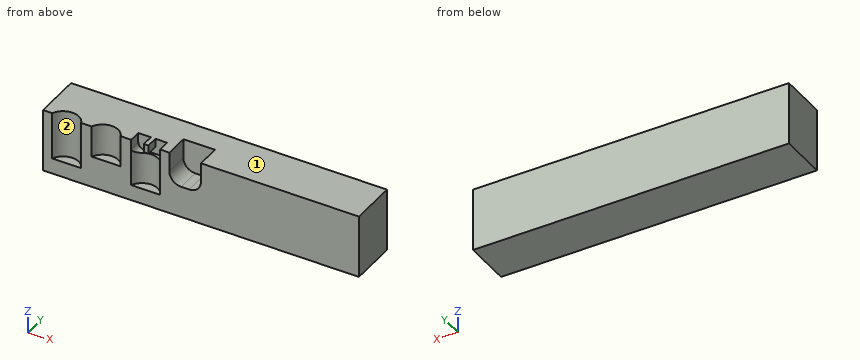
from build123d import *

# Parameters (mm, degrees)
F0_W      = 38.1
F0_H      = 50.8
F1_DEPTH  = 254
F3_DEPTH  = 38.1
F5_DEPTH  = 25.4
F7_DEPTH  = 38.1
F8_W      = 23.2794845304
F8_H      = 9.0677170083
F8_H_2    = 9.5680775121
F9_DEPTH  = 12.7
F10_R     = 5.08
F11_W     = 3.6223009229
F11_H     = 6.850992012
F12_DEPTH = 9.525
F14_DEPTH = 19.05
F15_R     = 9.525


with BuildPart() as f1:
    # F0 (on Right) → F1 (new body)
    with BuildSketch(Plane.YZ):
        with Locations((19.05, 25.4)):
            Rectangle(F0_W, F0_H)
    extrude(amount=F1_DEPTH)

    # F2 (on face) → F3 (cut)
    with BuildSketch(Plane.XY.offset(50.8)):
        with BuildLine():
            ThreePointArc((6.35, -5.08), (19.05, -17.78), (31.75, -5.08))
            ThreePointArc((31.75, -5.08), (19.05, 7.62), (6.35, -5.08))
        make_face()
    extrude(amount=-F3_DEPTH, mode=Mode.SUBTRACT)

    # F4 (on face) → F5 (cut)
    with BuildSketch(Plane.XY.offset(50.8)):
        with BuildLine():
            ThreePointArc((38.1, -5.08), (50.8, -17.78), (63.5, -5.08))
            ThreePointArc((63.5, -5.08), (50.8, 7.62), (38.1, -5.08))
        make_face()
    extrude(amount=-F5_DEPTH, mode=Mode.SUBTRACT)

    # F6 (on face) → F7 (cut)
    with BuildSketch(Plane.XY.offset(50.8)):
        with BuildLine():
            ThreePointArc((69.85, -5.08), (82.55, -17.78), (95.25, -5.08))
            ThreePointArc((95.25, -5.08), (82.55, 7.62), (69.85, -5.08))
        make_face()
    extrude(amount=-F7_DEPTH, mode=Mode.SUBTRACT)

    # F8 (on face) → F9 (cut)
    with BuildSketch(Plane.XY.offset(50.8)):
        with Locations((82.55, -4.5338585041)):
            Rectangle(F8_W, F8_H)
        with Locations((82.55, 4.784038756)):
            Rectangle(F8_W, F8_H_2)
    extrude(amount=-F9_DEPTH, mode=Mode.SUBTRACT)

    # F10
    f10_edges = [f1.edges().sort_by_distance(p)[0] for p in [
        (70.910258, 4.784039, 38.1),
        (94.189742, 4.784039, 38.1),
    ]]
    fillet(f10_edges, radius=F10_R)

    # F11 (on face) → F12 (join)
    with BuildSketch(Plane.XZ.offset(-9.5680775121)):
        with Locations((82.8721560538, 47.374503994)):
            Rectangle(F11_W, F11_H)
    extrude(amount=F12_DEPTH)

    # F13 (on face) → F14 (cut)
    with BuildSketch(Plane.XZ):
        Polygon((101.6, 50.8), (101.6, 38.1), (101.6, 25.4), (127, 25.4), (127, 50.8), align=None)
    extrude(amount=-F14_DEPTH, mode=Mode.SUBTRACT)

    # F15
    f15_edges = [f1.edges().sort_by_distance(p)[0] for p in [
        (101.6, 9.525, 25.4),
        (127, 9.525, 25.4),
    ]]
    fillet(f15_edges, radius=F15_R)


solid = f1.part
Geometry check sheet. Reference: the model listing, model coordinates, mm. Face numbers are marked on the shaded views. A direction names the side the tool comes from. Round coordinates to 2 decimals unless told otherwise and drop trailing zeros. Loops run counter-clockwise (first coordinate to the right, second up) from the corner with the lowest first, then second, coordinate; pieces in that order, holes last. Notation, with made-up numbers: (-11.5, 17) -> (32.5, 17) arc R18 ccw to (32.5, 48) -> close; hole circle Ø7 at (-31.5, 24.25). An arc over 180 degrees is marked (long way). Answer as a JSON object with one key per item and string values. Group by question number.
Item 1: Set-up check for the marked faces 1 and 2: record each of +Z, -Z, +X, -X, +Y, -Y from which the full face is reachable in a straight line by a thin tool's end or side.
Item 2: Thickness scan on line 1 along Y through (x, z) = (121, 32.5); line 2 along Y through (x, z) = (61, 40); line 3 along Z through (x, y) = (122, 10). Record the ranges inside material, lowest first.
Item 3: Cross-section at A-A, the plane z = 20. Record the cut outline in (x, y), plus the area to 3 significant figures.
Item 4: Cross-section at C-C, the plane z = 30.5. Record the cut outline in (x, y), plus the area to 3 significant figures.
Item 5: Depth check by flat-ended pin: pin 1 Ø20.5 at (x, z) = (120.5, 44) entering from -Y; pin 2 Ø6 at (x, y) = (18, 3) entering from +Z; pin 3 Ø6 at (x, y) = (56.5, 2) entering from +Z; pin 4 Ø1.5 at (x, z) = (72.5, 45.5) entering from -Y. Enter the tip coordinate at first touch or a pass-through.
Item 6: Cross-section at B-B, the plane y = 12.5. Record the cut outline in (x, z) (3 decimals), plus the area to 3 significant figures.
Determined:
{
 "1": {"face 1": "+Z, +X, -X, +Y, -Y", "face 2": "+Z, -Y"},
 "2": {"line 1": "y = 19.05 to 38.1", "line 2": "y = 2.49 to 38.1", "line 3": "z = 0 to 26.54"},
 "3": {"outline": "(0, 0) -> (7.41, 0) arc R12.7 cw to (30.69, 0) -> (70.91, 0) arc R12.7 cw to (94.19, 0) -> (254, 0) -> (254, 38.1) -> (0, 38.1) -> close", "area": "9,420 mm²"},
 "4": {"outline": "(0, 0) -> (7.41, 0) arc R12.7 cw to (30.69, 0) -> (39.16, 0) arc R12.7 cw to (62.44, 0) -> (70.91, 0) arc R12.7 cw to (94.19, 0) -> (102.69, 0) -> (102.69, 19.05) -> (125.91, 19.05) -> (125.91, 0) -> (254, 0) -> (254, 38.1) -> (0, 38.1) -> close", "area": "8,850 mm²"},
 "5": {"pin 1": "stops at y = 0", "pin 2": "stops at z = 12.7", "pin 3": "stops at z = 25.4", "pin 4": "stops at y = 9.57"},
 "6": {"outline": "(0, 0) -> (254, 0) -> (254, 50.8) -> (127, 50.8) -> (127, 34.925) arc R9.525 cw to (117.475, 25.4) -> (111.125, 25.4) arc R9.525 cw to (101.6, 34.925) -> (101.6, 50.8) -> (0, 50.8) -> close", "area": "12,300 mm²"}
}
